Can you work these out from the model? Positions are in its coordinate system, mm. Face numbers are marked on the shaded views. A direction names the side the tool comes from. Give positions to 0.01 mm unless a question says otherwise; leave off trailing zeros. Order: outer loops, then holes, each group sorted by start corner. A loop starts at its lowest first (then second) coordinate and runs counter-clockwise, first axis right, second up. Notation, with made-up numbers: M 79,14 L 102,14 A13 cw 102,18 Z; hole C 60.5,-29 d10. An arc over 180 degrees is marked long. One line per question, with ' | ' between items. Start each with the question number.
1) If we section it at B-B, the plane z = 8: State how many separate pieces and enclosed holes the cut face has, plus the area to 3 significant figures.
2) For the marked faces 1 and 2, which set-ups out of +Z, -Z, +X, -X, +Y, -Y let a thin tool reach every point of the face, with its end or its side?
3) I'm going to push a flat-ended pin straight in: pin 1 Ø1 at (x, y) = (6.5, 119.5) entering from +Z. Where does the tip first touch, or does it pass through?
4) If we section it at A-A, the plane y = -127: Please give me the cut outline in (x, z), plus the area to 3 significant figures.
5) Please list where these lines run through material, in increasing order: line 1 along Y through (x, z) = (-24, 29); line 2 along X through (y, z) = (125, 17); line 3 along Y through (x, z) = (7, 23). Write a range as [from, to].
6) Thinking about a two-plate mould opening in X: for the marked faces 3, 4 and 5, which applies, +X half, -X half, draft (parallel to the pull), parting line (faces both ways), or undercut?
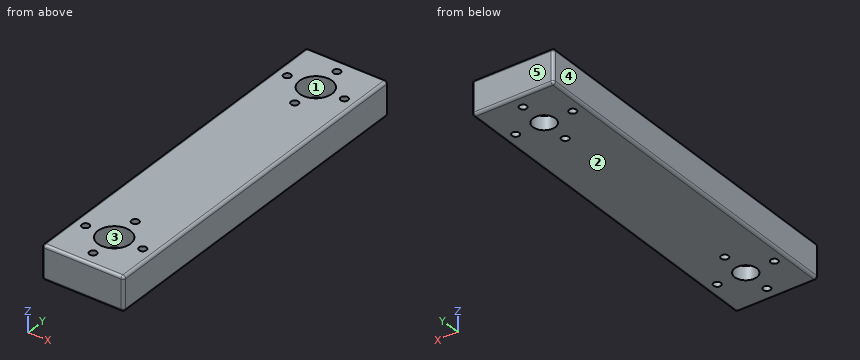
```python
from build123d import *

# Parameters (mm, degrees)
SKETCH1_W           = 333.502
SKETCH1_H           = 76.2
BOSS_EXTRUDE1_DEPTH = 31.75
SKETCH2_R           = 15.113
CUT_EXTRUDE1_DEPTH  = 19.05
SKETCH3_R           = 10.287
CUT_EXTRUDE2_DEPTH  = 173.105806122
SKETCH4_R           = 3.429
CUT_EXTRUDE3_DEPTH  = 174.970021846
FILLET1_R           = 2.54


with BuildPart() as part:
    # Sketch1 → Boss-Extrude1 (new body)
    with BuildSketch(Plane(origin=(0, 0, 0), x_dir=(0, 1, 0), z_dir=(0, 0, 1))):
        Rectangle(SKETCH1_W, SKETCH1_H)
    extrude(amount=BOSS_EXTRUDE1_DEPTH)

    # Sketch2 → Cut-Extrude1 (cut)
    with BuildSketch(Plane.XY.offset(31.75)):
        with Locations((0, 127)):
            Circle(SKETCH2_R)
        with Locations((0, -127)):
            Circle(SKETCH2_R)
    extrude(amount=-CUT_EXTRUDE1_DEPTH, mode=Mode.SUBTRACT)

    # Sketch3 → Cut-Extrude2 (cut, through all)
    with BuildSketch(Plane.XY.offset(12.7)):
        with Locations((0, -127)):
            Circle(SKETCH3_R)
        with Locations((0, 127)):
            Circle(SKETCH3_R)
    extrude(amount=-CUT_EXTRUDE2_DEPTH, mode=Mode.SUBTRACT)

    # Sketch4 → Cut-Extrude3 (cut, through all)
    with BuildSketch(Plane.XY.offset(31.75)):
        with Locations((-26.543, 127)):
            Circle(SKETCH4_R)
        with Locations((0, 153.543)):
            Circle(SKETCH4_R)
        with Locations((26.543, 127)):
            Circle(SKETCH4_R)
        with Locations((0, 100.457)):
            Circle(SKETCH4_R)
        with Locations((0, -100.457)):
            Circle(SKETCH4_R)
        with Locations((26.543, -127)):
            Circle(SKETCH4_R)
        with Locations((0, -153.543)):
            Circle(SKETCH4_R)
        with Locations((-26.543, -127)):
            Circle(SKETCH4_R)
    extrude(amount=-CUT_EXTRUDE3_DEPTH, mode=Mode.SUBTRACT)

    # Fillet1
    fillet1_edges = [part.edges().sort_by_distance(p)[0] for p in [
        (0, -166.751, 31.75),
        (38.1, 0, 31.75),
        (0, 166.751, 31.75),
        (38.1, 0, 0),
        (0, -166.751, 0),
        (-38.1, 0, 0),
        (0, 166.751, 0),
        (38.1, 166.751, 15.875),
        (38.1, -166.751, 15.875),
        (-38.1, -166.751, 15.875),
        (-38.1, 166.751, 15.875),
        (-38.1, 0, 31.75),
    ]]
    fillet(fillet1_edges, radius=FILLET1_R)


solid = part.part
```
Results found:
1) separate pieces: 1 | enclosed holes: 10 | area: 24,400 mm²
2) face 1: +Z | face 2: -Z, +X, -X, +Y, -Y
3) pin 1: stops at z = 12.7
4) outline: M -38.1,2.54 A2.54 ccw -35.56,0 L -29.97,0 L -29.97,31.75 L -35.56,31.75 A2.54 ccw -38.1,29.21 Z; M -23.11,0 L -10.29,0 L -10.29,12.7 L -15.11,12.7 L -15.11,31.75 L -23.11,31.75 Z; M 10.29,0 L 23.11,0 L 23.11,31.75 L 15.11,31.75 L 15.11,12.7 L 10.29,12.7 Z; M 29.97,0 L 35.56,0 A2.54 ccw 38.1,2.54 L 38.1,29.21 A2.54 ccw 35.56,31.75 L 29.97,31.75 Z | area: 1,140 mm²
5) line 1: y = [-166.75, -129.3], [-124.7, 124.7], [129.3, 166.75] | line 2: x = [-38.1, -29.33], [-23.76, -14.98], [14.98, 23.76], [29.33, 38.1] | line 3: y = [-166.75, -140.39], [-113.61, 113.61], [140.39, 166.75]
6) face 3: undercut | face 4: -X half | face 5: draft
